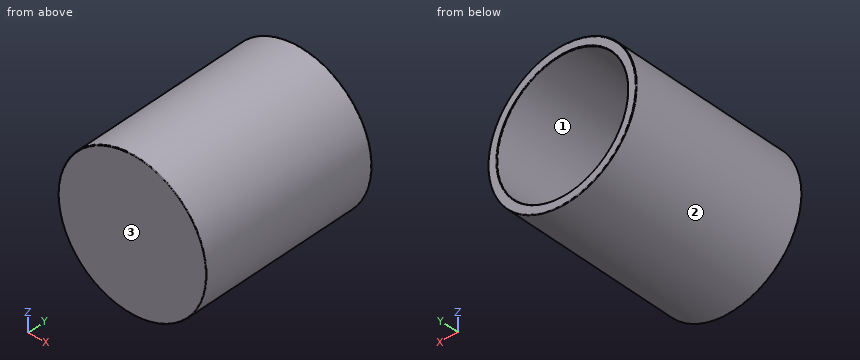
from build123d import *


with BuildPart() as f1:
    # F0 (on Top) → F1 (revolve)
    with BuildSketch(Plane.XY):
        with BuildLine():
            Line((0, -25.1593), (0, -20))
            Line((0, -20), (-36.3407, -20))
            ThreePointArc((-36.3407, -20), (-38.815574, -18.974874), (-39.8407, -16.5))
            Line((-39.8407, -16.5), (-39.8407, 84.8093))
            ThreePointArc((-39.8407, 84.8093), (-39.943213, 85.056787), (-40.1907, 85.1593))
            Line((-40.1907, 85.1593), (-44.65, 85.1593))
            ThreePointArc((-44.65, 85.1593), (-44.897487, 85.056787), (-45, 84.8093))
            Line((-45, 84.8093), (-45, -24.8093))
            ThreePointArc((-45, -24.8093), (-44.897487, -25.056787), (-44.65, -25.1593))
            Line((-44.65, -25.1593), (0, -25.1593))
        make_face()
    revolve(axis=Axis((0, -25.1593, 0), (0, -1, 0)))


solid = f1.part
Verification items for the finished model (mm, model axes). Face numbers are marked on the shaded views. Round coordinates to 2 decimals unless told otherwise and drop trailing zeros. Order: outer loops, then holes, each group sorted by start corner. A loop starts at its lowest first (then second) coordinate and runs counter-clockwise, first axis right, second up. Notation, with made-up numbers: (88, 14.5) -> (129, 14.5) arc R29 ccw to (129, 53.5) -> close; hole circle Ø5 at (43.5, -9). An arc over 180 degrees is marked (long way). Put each result on its own line as item: value.
1) Section check A-A (z = 0). Record the cut outline in (x, y).
Final values:
outline: (-45, -24.81) arc R0.35 ccw to (-44.65, -25.16) -> (44.65, -25.16) arc R0.35 ccw to (45, -24.81) -> (45, 84.81) arc R0.35 ccw to (44.65, 85.16) -> (40.19, 85.16) arc R0.35 ccw to (39.84, 84.81) -> (39.84, -16.5) arc R3.5 cw to (36.34, -20) -> (-36.34, -20) arc R3.5 cw to (-39.84, -16.5) -> (-39.84, 84.81) arc R0.35 ccw to (-40.19, 85.16) -> (-44.65, 85.16) arc R0.35 ccw to (-45, 84.81) -> close
2) Section check D-D (y = -18). Record the cut outline in (x, z).
Final values:
outline: circle Ø90 at (0, 0); hole circle Ø79.01 at (0, 0)
3) Section check C-C (y = 34). Record the cut outline in (x, z), then the cut area to 3 significant figures.
Final values:
outline: circle Ø90 at (0, 0); hole circle Ø79.68 at (0, 0)
area: 1,380 mm^2
4) Section check B-B (x = 0). Record the cut outline in (y, z).
Final values:
outline: (-25.16, -44.65) arc R0.35 ccw to (-24.81, -45) -> (84.81, -45) arc R0.35 ccw to (85.16, -44.65) -> (85.16, -40.19) arc R0.35 ccw to (84.81, -39.84) -> (-16.5, -39.84) arc R3.5 cw to (-20, -36.34) -> (-20, 36.34) arc R3.5 cw to (-16.5, 39.84) -> (84.81, 39.84) arc R0.35 ccw to (85.16, 40.19) -> (85.16, 44.65) arc R0.35 ccw to (84.81, 45) -> (-24.81, 45) arc R0.35 ccw to (-25.16, 44.65) -> close
5) Depth check by flat-ended pin: pin 1 (4 mm diameter, centred on y = 2.5, z = -23.5, fed in from +X); pin 2 (10 mm diameter, centred on x = -23.5, z = -27, fed in from +Y); pin 3 (8 mm diameter, centred on x = 11.5, y = 63, fed in from +Z); pin 4 (12 mm diameter, centred on x = 6.5, y = 13, fed in from +Z). Enter the tip coordinate at first touch or a pass-through.
Final values:
pin 1: stops at x = 39.53
pin 2: stops at y = 85.16
pin 3: stops at z = 44.37
pin 4: stops at z = 45
6) Mould release check, pull along Z, two halves, no side actions. Record for the marked faces 1, 2 and 3: +Z half, -Z half, draft (parallel to the pull), parting line (faces both ways), or undercut.
Final values:
face 1: undercut
face 2: parting line
face 3: draft
7) Material ranges on line 1 (X direction, y = 39, z = 0); line 2 (X direction, y = -18.5, z = 14), recorded low to high.
Final values:
line 1: x = -45 to -39.84, 39.84 to 45
line 2: x = -42.77 to -36.63, 36.63 to 42.77
